Read the model definition and answer for the solid it produces. Units are mm, in the model's axes. Give positions to 0.01 mm unless a question says otherwise; leave off trailing zeros. Order: outer loops, then holes, each group sorted by start corner. A loop starts at its lowest first (then second) coordinate and runs counter-clockwise, first axis right, second up. Notation, with made-up numbers: (1.25, 49) - (43.25, 49) arc R35 ccw to (43.25, 88) - close; hole circle Ø7 at (49, -36). An arc over 180 degrees is marked (long way). Write each question's results on one line, items separated by ' | '.
from build123d import *

# Parameters (mm, degrees)
SKETCH1_R           = 20
BOSS_EXTRUDE1_DEPTH = 1
DOME1_FACE_RADIUS   = 20
DOME1_HEIGHT        = 20
SKETCH2_R           = 5
BOSS_EXTRUDE2_DEPTH = 20
SKETCH3_R           = 18.75
BOSS_EXTRUDE3_DEPTH = 1


# Read off the part's stored shape, not the designer's step: Shell1
with BuildPart() as part:
    # Sketch1 → Boss-Extrude1 (new body)
    with BuildSketch(Plane.XY):
        with Locations((-47.148513575, 20.745345973)):
            Circle(SKETCH1_R)
    extrude(amount=BOSS_EXTRUDE1_DEPTH)

    # Dome1: a dome of height H over a round flat face of radius A is a cap of a sphere of radius (A * A + H * H) / (2 * H)
    dome1_r = (DOME1_FACE_RADIUS * DOME1_FACE_RADIUS + DOME1_HEIGHT * DOME1_HEIGHT) / (2 * DOME1_HEIGHT)
    dome1_base = Plane((-47.148513575, 20.745345973, 1), z_dir=(0, 0, 1))
    with Locations(dome1_base.offset(DOME1_HEIGHT - dome1_r)):
        dome1_ball = Sphere(dome1_r, mode=Mode.PRIVATE)
    add(split(dome1_ball, bisect_by=dome1_base, keep=Keep.TOP, mode=Mode.PRIVATE))

    # Shell1 outline → Shell1 (revolve, cut)
    with BuildSketch(Plane(origin=(-47.148513575, 20.745345973, 0), x_dir=(1, 0, 0), z_dir=(0, -1, 0))):
        with BuildLine():
            Line((17, 0), (17, 0.999999983))
            ThreePointArc((17, 0.999999983), (12.020815286, 13.020815274), (0, 18))
            Line((0, 18), (0, 0))
            Line((0, 0), (17, 0))
        make_face()
    revolve(axis=Axis((-47.148513575, 20.745345973, 0), (0, 0, 1)), mode=Mode.SUBTRACT)

    # Sketch2 → Boss-Extrude2 (add)
    with BuildSketch(Plane(origin=(0, 0, 0), x_dir=(-1, 0, 0), z_dir=(0, 0, -1))):
        with Locations((47.148513575, 20.745345973)):
            Circle(SKETCH2_R)
    extrude(amount=-BOSS_EXTRUDE2_DEPTH)

    # Sketch3 → Boss-Extrude3 (add)
    with BuildSketch(Plane(origin=(0, 0, 0), x_dir=(-1, 0, 0), z_dir=(0, 0, -1))):
        with Locations((47.148513575, 20.745345973)):
            Circle(SKETCH3_R)
    extrude(amount=-BOSS_EXTRUDE3_DEPTH)


solid = part.part
(1) Consider probe 1 along Y at (x, z) = (-46, 6.5); probe 2 along Y at (x, z) = (-43.5, 5); probe 3 along X at (y, z) = (20.5, 8.5). Determine where each line is inside the solid, lowest interval first. Write a range as [from, to].
Conclusion:
probe 1: [1.55, 4.7], [15.88, 25.61], [36.79, 39.94] | probe 2: [1.49, 4.63], [17.33, 24.16], [36.86, 40] | probe 3: [-65.69, -62.4], [-52.14, -42.15], [-31.89, -28.61]
(2) Section D-D (y = 19) is taken. Give the vertices of the cut face in (x, z), plus the area to 3 significant figures.
Conclusion:
outline: (-67.07, 0) - (-27.22, 0) - (-27.22, 1) arc R19.92 ccw to (-67.07, 1) - close; hole (-64.06, 1) - (-51.83, 1) - (-51.83, 17.25) arc R16.91 ccw to start; hole (-42.46, 1) - (-30.24, 1) arc R16.91 ccw to (-42.46, 17.25) - close | area: 371 mm^2
(3) Section C-C (y = 34.5) is taken. Give the vertices of the cut face in (x, z), plus the area to 3 significant figures.
Conclusion:
outline: (-61.67, 0) - (-32.63, 0) - (-32.63, 1) arc R14.52 ccw to (-61.67, 1) - close; hole (-57.14, 1) - (-37.16, 1) arc R9.99 ccw to start | area: 203 mm^2
(4) The mould has two halves that part along X. Classify faces 1 (the face through (-28.67, 13.09, 0.49)), 2 (the face through (-47, 21, 0)), 3 (the face through (-49.46, 16.31, 9.01)): pulls with the +X half, pulls with the -X half, needs draft (parallel to the pull), parting line crosses it, or undercut.
Conclusion:
face 1: parting line crosses it | face 2: needs draft | face 3: undercut
(5) Section B-B (z = 3.5) is taken. Give the vertices of the cut face in (x, y).
Conclusion:
outline: circle Ø39.69 at (-47.15, 20.75); circle Ø10 at (-47.15, 20.75); hole circle Ø33.63 at (-47.15, 20.75)
(6) Each of these flat-tipped pins is pushed along its axis until it touches: pin 1 (1.5 mm diameter, centred on x = -57, y = 23.5, fed in from +Z); pin 2 (6 mm diameter, centred on x = -47, z = 6, fed in from +Y); pin 3 (10 mm diameter, centred on x = -34.5, y = 12.5, fed in from +Z); pin 4 (1 mm diameter, centred on y = 6, z = 15.5, fed in from -X). Where does it stop, or does it pass through?
Conclusion:
pin 1: z = 18.61 | pin 2: y = 40.64 | pin 3: z = 18.26 | pin 4: through
